from build123d import *

# Parameters (mm, degrees)
SKETCH3_W           = 7.5
SKETCH3_H           = 6.25
SKETCH3_R           = 0.9
BOSS_EXTRUDE1_DEPTH = 2
SKETCH6_R           = 0.9
BOSS_EXTRUDE3_DEPTH = 1.85


with BuildPart() as part:
    # Sketch3 → Boss-Extrude1 (new body)
    with BuildSketch(Plane(origin=(0, 0, 0), x_dir=(1, 0, 0), z_dir=(0, 1, 0))):
        with Locations((1.25, 0)):
            Rectangle(SKETCH3_W, SKETCH3_H)
        with Locations(Location((0, 0, 0), (0, 0, 270))):
            Circle(SKETCH3_R, mode=Mode.SUBTRACT)
    extrude(amount=BOSS_EXTRUDE1_DEPTH)

    # Sketch6 → Boss-Extrude3 (add)
    with BuildSketch(Plane(origin=(0, 2, 0), x_dir=(1, 0, 0), z_dir=(0, 1, 0))):
        with BuildLine():
            Line((-2.5, 3.125), (-2.5, -3.125))
            Line((-2.5, -3.125), (1.953229167, -3.125))
            ThreePointArc((1.953229167, -3.125), (1.5, 0), (1.953229167, 3.125))
            Line((1.953229167, 3.125), (-2.5, 3.125))
        make_face()
        with Locations(Location((0, 0, 0), (0, 0, 270))):
            Circle(SKETCH6_R, mode=Mode.SUBTRACT)
    extrude(amount=BOSS_EXTRUDE3_DEPTH)


solid = part.part
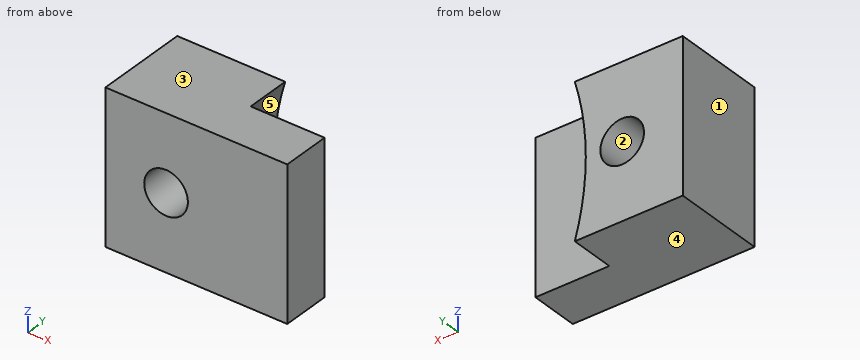
Input: part model. Units: mm. Frame: model coordinates. Face numbers are marked on the shaded views. A direction names the side the tool comes from. Round coordinates to 2 decimals unless told otherwise and drop trailing zeros. Order: outer loops, then holes, each group sorted by start corner. A loop starts at its lowest first (then second) coordinate and runs counter-clockwise, first axis right, second up. Notation, with made-up numbers: (57, 74.5) - (91, 74.5) arc R18 ccw to (91, 96.5) - close; hole circle Ø8 at (-5, -14). An arc over 180 degrees is marked (long way). Answer as a JSON object with one key per item and string values. Group by question number.
(1) Pin query (flat end, axial travel): P1, Ø3, axis at x = 2, z = -2, coming from the -Y side; P2, Ø1.1, axis at x = 3, z = 0.5, coming from the +Y side. Return the tip coordinate at first contact, or that it passes through.
(2) Draft query along Z for the marked faces 1, 2 and 3. Return one class per face: released by +Z, released by -Z, zero draft, split by the parting line, or undercut.
(3) Cut plane C-C (y = 0.45). Return loops of the section in (x, z) (3 decimals).
(4) Cut plane D-D (y = 2.45). Return loops of the section in (x, z) (3 decimals), then the cut area to 3 significant figures.
(5) Cut plane B-B (x = 0). Return loops of the section in (y, z) (3 decimals).
(6) Cut plane A-A (z = 0). Return loops of the section in (x, y).
(7) Material intervals for probe 1 along X at (y, z) = (2.35, 0); probe 2 along Y at (x, z) = (3, 0.25); probe 3 along X at (y, z) = (3.7, 0.5), sorted ascending. Write a range as from..to.
(8) Reachability of the marked faces 4 and 5 from +Z, -Z, +X, -X, +Y, -Y: full face, straight path, thin tool, end or side. Return the list, or none.
Here are the results:
{
 "1": {"P1": "stops at y = 0", "P2": "stops at y = 2"},
 "2": {"face 1": "zero draft", "face 2": "undercut", "face 3": "released by +Z"},
 "3": {"outline": "(-2.5, -3.125) - (5, -3.125) - (5, 3.125) - (-2.5, 3.125) - close; hole circle Ø1.8 at (0, 0)"},
 "4": {"outline": "(-2.5, -3.125) - (1.953, -3.125) arc R11 cw to (1.953, 3.125) - (-2.5, 3.125) - close; hole circle Ø1.8 at (0, 0)", "area": "23.4 mm^2"},
 "5": {"outline": "(0, -3.125) - (3.85, -3.125) - (3.85, -0.9) - (0, -0.9) - close; (0, 0.9) - (3.85, 0.9) - (3.85, 3.125) - (0, 3.125) - close"},
 "6": {"outline": "(-2.5, 0) - (-0.9, 0) - (-0.9, 3.85) - (-2.5, 3.85) - close; (0.9, 0) - (5, 0) - (5, 2) - (1.5, 2) - (1.5, 3.85) - (0.9, 3.85) - close"},
 "7": {"probe 1": "x = -2.5..-0.9, 0.9..1.5", "probe 2": "y = 0..2", "probe 3": "x = -2.5..-0.75, 0.75..1.51"},
 "8": {"face 4": "-Z, +X, -X, +Y, -Y", "face 5": "+X, +Y"}
}
